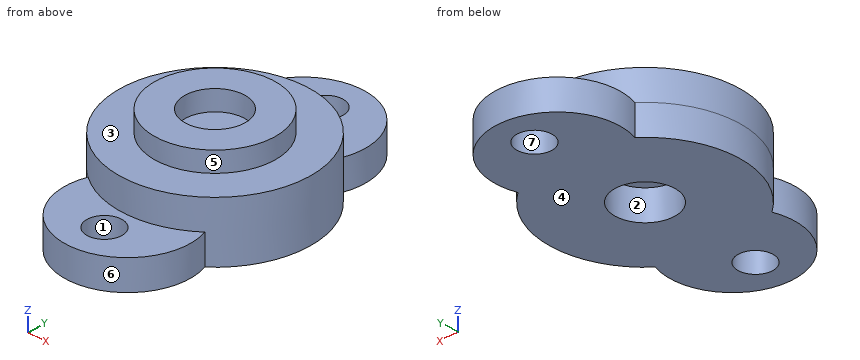
```python
from build123d import *

# Parameters (mm, degrees)
SKETCH1_R      = 12
SKETCH1_R_2    = 3.5
EXTRUDE1_DEPTH = 6
SKETCH1_3_R    = 12
SKETCH1_3_R_2  = 6
EXTRUDE2_DEPTH = 16
SKETCH2_R      = 19
EXTRUDE3_DEPTH = 6


with BuildPart() as part:
    # Sketch1 → Extrude1 (new body)
    with BuildSketch(Plane.XY):
        with BuildLine():
            ThreePointArc((11.804353201, 14.888157895), (0, 31.5), (-11.804353201, 14.888157895))
            ThreePointArc((-11.804353201, 14.888157895), (-19, 0), (-11.804353201, -14.888157895))
            ThreePointArc((-11.804353201, -14.888157895), (0, -31.5), (11.804353201, -14.888157895))
            ThreePointArc((11.804353201, -14.888157895), (19, 0), (11.804353201, 14.888157895))
        make_face()
        Circle(SKETCH1_R, mode=Mode.SUBTRACT)
        with Locations((0, 24)):
            Circle(SKETCH1_R_2, mode=Mode.SUBTRACT)
        with Locations((0, -24)):
            Circle(SKETCH1_R_2, mode=Mode.SUBTRACT)
    extrude(amount=EXTRUDE1_DEPTH)

    # Sketch1<3> → Extrude2 (add)
    with BuildSketch(Plane.XY):
        Circle(SKETCH1_3_R)
        Circle(SKETCH1_3_R_2, mode=Mode.SUBTRACT)
    extrude(amount=EXTRUDE2_DEPTH)

    # Sketch2 → Extrude3 (add)
    with BuildSketch(Plane.XY.offset(6)):
        Circle(SKETCH2_R)
    extrude(amount=EXTRUDE3_DEPTH)


solid = part.part
```
Part model, mm, in its own coordinate system. Face numbers are marked on the shaded views. A direction names the side the tool comes from. Round coordinates to 2 decimals unless told otherwise and drop trailing zeros. Loops run counter-clockwise (first coordinate to the right, second up) from the corner with the lowest first, then second, coordinate; pieces in that order, holes last. Notation, with made-up numbers: (32.5, 13) -> (81.5, 13) arc R12 ccw to (81.5, 26) -> close; hole circle Ø3 at (-19.5, 51). An arc over 180 degrees is marked (long way). Use one line per item in the form item = value. Start each with the question number.
Item 1: Band-saw the part on A-A (x = 0). List the corners of the cut face in (y, z).
Item 2: Band-saw the part on D-D (z = 9). List the corners of the cut face in (x, y).
Item 3: Tool access for the marked faces 1, 2 and 3: list every direction of +Z, -Z, +X, -X, +Y, -Y with a clear straight run to the whole face (end or side of a thin tool).
Item 4: Band-saw the part on B-B (z = 2.25). List the corners of the cut face in (x, y), plus the area to 3 significant figures.
Item 5: Band-saw the part on C-C (y = 24). List the corners of the cut face in (x, z), plus the area to 3 significant figures.
Item 6: Drop flat-ended pins along their axis: pin 1 Ø2 at (x, z) = (-10, 9.5) entering from +Y; pin 2 Ø11 at (x, y) = (0, -24) entering from +Z; pin 3 Ø2 at (x, z) = (-5, 14) entering from -Y. Give the stop position or say it passes through.
Item 7: Drill centre lines: line 1 along Y through (x, z) = (0, 14.6); line 2 along X through (y, z) = (0, 4.05); line 3 along Z through (x, y) = (-9, -17.5). Where is each one in solid material? Low to high.
Item 8: Two-plate mould, pull along Y, no slides. Class the marked faces 4, 5, 6 and 7: released by +Y, released by -Y, zero draft, split by the parting line, or undercut.
Data:
q1.outline = (-31.5, 0) -> (-27.5, 0) -> (-27.5, 6) -> (-31.5, 6) -> close; (-20.5, 0) -> (-6, 0) -> (-6, 6) -> (6, 6) -> (6, 0) -> (20.5, 0) -> (20.5, 6) -> (19, 6) -> (19, 12) -> (12, 12) -> (12, 16) -> (6, 16) -> (6, 12) -> (-6, 12) -> (-6, 16) -> (-12, 16) -> (-12, 12) -> (-19, 12) -> (-19, 6) -> (-20.5, 6) -> close; (27.5, 0) -> (31.5, 0) -> (31.5, 6) -> (27.5, 6) -> close
q2.outline = circle Ø38 at (0, 0)
q3.face_1 = +Z, -Z
q3.face_2 = -Z
q3.face_3 = +Z
q4.outline = (-11.8, -14.89) arc R12.5 ccw (long way) to (11.8, -14.89) arc R19 ccw to (11.8, 14.89) arc R12.5 ccw (long way) to (-11.8, 14.89) arc R19 ccw to start; hole circle Ø12 at (0, 0); hole circle Ø7 at (0, -24); hole circle Ø7 at (0, 24)
q4.area = 1,500 mm^2
q5.outline = (-11.46, 0) -> (-3.5, 0) -> (-3.5, 6) -> (-11.46, 6) -> close; (3.5, 0) -> (11.46, 0) -> (11.46, 6) -> (3.5, 6) -> close
q5.area = 95.5 mm^2
q6.pin_1 = 16.73
q6.pin_2 = 12
q6.pin_3 = -11.31
q7.line_1 = -12 to -6, 6 to 12
q7.line_2 = -19 to -6, 6 to 19
q7.line_3 = 0 to 6
q8.face_4 = zero draft
q8.face_5 = split by the parting line
q8.face_6 = undercut
q8.face_7 = undercut
